Can you work these out from the model? Positions are in its coordinate system, mm. Round coordinates to 2 decimals unless told otherwise and drop trailing zeros. Write each loop counter-clockwise with the first axis right and the second up, starting at its lowest first coordinate (ties: lowest second). Pieces come first, ordered by that corner, then holes. Notation, with made-up numbers: M -11.75,32 L 20.25,32 A19 ccw 20.25,54 Z; hole C -23.75,-36.75 d1. An arc over 180 degrees is marked long. Answer as a JSON object with one key per item and string values. Group by question number.
1) Please list where these lines run through material, in increasing order: L1, parallel to X at y = 8, z = -269; L2, parallel to X at y = 4.25, z = 182; L3, parallel to Z at x = 49, y = 14.75. Write a range as [from, to].
2) Suppose I cut it at A-A, the plane z = -158.5. Write out the boundary of the cut face in (x, y), and give its area (3 significant figures).
3) I'm going to push flat-ended pins straight in: pin 1 Ø8 at (y, z) = (3, -287.5) entering from +X; pin 2 Ø3 at (x, y) = (-46, 12) entering from -Z. Where does each tip first touch, or does it pass through?
from build123d import *

# Parameters (mm, degrees)
SKETCH1_W           = 1750
SKETCH1_H           = 895
BOSS_EXTRUDE1_DEPTH = 20
SKETCH2_W           = 210
SKETCH2_H           = 660
CUT_EXTRUDE1_DEPTH  = 20
FILLET1_R           = 5


with BuildPart() as part:
    # Sketch1 → Boss-Extrude1 (new body)
    with BuildSketch(Plane(origin=(0, 0, 0), x_dir=(1, 0, 0), z_dir=(0, 1, 0))):
        Rectangle(SKETCH1_W, SKETCH1_H)
    extrude(amount=BOSS_EXTRUDE1_DEPTH)

    # Sketch2 → Cut-Extrude1 (cut)
    with BuildSketch(Plane(origin=(0, 20, 0), x_dir=(1, 0, 0), z_dir=(0, 1, 0))):
        with Locations((0, 447.5)):
            Rectangle(SKETCH2_W, SKETCH2_H)
    extrude(amount=-CUT_EXTRUDE1_DEPTH, mode=Mode.SUBTRACT)

    # Fillet1
    fillet1_edges = [part.edges().sort_by_distance(p)[0] for p in [
        (-875, 20, 0),
        (-490, 0, -447.5),
        (-105, 0, -282.5),
        (-490, 20, -447.5),
        (0, 20, 447.5),
        (105, 20, -282.5),
        (-105, 20, -282.5),
        (0, 20, -117.5),
        (105, 0, -282.5),
        (105, 10, -447.5),
        (-105, 10, -447.5),
        (-105, 10, -117.5),
        (0, 0, -117.5),
        (105, 10, -117.5),
        (875, 20, 0),
        (0, 0, 447.5),
        (-875, 0, 0),
        (490, 0, -447.5),
        (875, 0, 0),
        (875, 10, 447.5),
        (-875, 10, 447.5),
        (-875, 10, -447.5),
        (875, 10, -447.5),
        (490, 20, -447.5),
    ]]
    fillet(fillet1_edges, radius=FILLET1_R)


solid = part.part
Results:
{
 "1": {"L1": "[-875, -105], [105, 875]", "L2": "[-874.94, 874.94]", "L3": "[-117.5, 447.5]"},
 "2": {"outline": "M -875,5 A5 ccw -870,0 L -110,0 A5 ccw -105,5 L -105,15 A5 ccw -110,20 L -870,20 A5 ccw -875,15 Z; M 105,5 A5 ccw 110,0 L 870,0 A5 ccw 875,5 L 875,15 A5 ccw 870,20 L 110,20 A5 ccw 105,15 Z", "area": "30,800 mm^2"},
 "3": {"pin 1": "x = 875", "pin 2": "z = -117.5"}
}
